Verification items for the finished model (mm, model axes). A direction names the side the tool comes from. Give positions to 0.01 mm unless a question says otherwise; leave off trailing zeros. Loops run counter-clockwise (first coordinate to the right, second up) from the corner with the lowest first, then second, coordinate; pieces in that order, holes last. Notation, with made-up numbers: M 19,31 L 76,31 A19 ccw 76,48 Z; hole C 82.5,18.5 d7. An arc over 180 degrees is marked long. Answer in a Markdown table with one row per item.
```python
from build123d import *

# Parameters (mm, degrees)
BOSS_EXTRUDE1_DEPTH         = 25.4
F_1_4_0_25_DIAMETER_HOLE1_D = 6.35


with BuildPart() as part:
    # Sketch1 → Boss-Extrude1 (new body)
    with BuildSketch(Plane(origin=(0, 0, 0), x_dir=(1, 0, 0), z_dir=(0, 1, 0))):
        Polygon((67.945, 0), (85.09, 0), (85.09, -5.08), (0, -5.08), (0, 0), (17.145, 0), (17.145, 5.08), (67.945, 5.08), align=None)
    extrude(amount=BOSS_EXTRUDE1_DEPTH)

    # 1/4 (0.25) Diameter Hole1 (through all)
    with Locations(Plane.XY.offset(5.08)):
        with Locations((5.715, 12.7), (79.375, 12.7)):
            Hole(F_1_4_0_25_DIAMETER_HOLE1_D / 2)


solid = part.part
```
Item 1: Scan lines: L1, parallel to X at y = 13.5, z = 1; L2, parallel to X at y = 14.5, z = -4.5 (3 decimals); L3, parallel to Z at x = 17, y = 15. Record each from-to range of solid material in increasing order. Write a range as [from, to].
Reported:
| item | result |
|---|---|
| L1 | x = [0, 2.64], [8.79, 76.3], [82.45, 85.09] |
| L2 | x = [17.145, 67.945] |
| L3 | z = [0, 5.08] |
Item 2: Sectioned sample at B-B (z = 1.5). Record the cut outline in (x, y) (3 decimals).
Reported:
| item | result |
|---|---|
| outline | M 0,0 L 85.09,0 L 85.09,25.4 L 0,25.4 Z; hole C 5.715,12.7 d6.35; hole C 79.375,12.7 d6.35 |
Item 3: Sectioned sample at D-D (x = 15). Record the cut outline in (y, z), and give its area (3 significant figures).
Reported:
| item | result |
|---|---|
| outline | M 0,0 L 25.4,0 L 25.4,5.08 L 0,5.08 Z |
| area | 129 mm^2 |
Item 4: Sectioned sample at A-A (y = 12.7). Record the cut outline in (x, z) (3 decimals), and give its area (3 significant figures).
Reported:
| item | result |
|---|---|
| outline | M 0,0 L 2.54,0 L 2.54,5.08 L 0,5.08 Z; M 8.89,0 L 17.145,0 L 17.145,-5.08 L 67.945,-5.08 L 67.945,0 L 76.2,0 L 76.2,5.08 L 8.89,5.08 Z; M 82.55,0 L 85.09,0 L 85.09,5.08 L 82.55,5.08 Z |
| area | 626 mm^2 |
Item 5: Go/stop test with flat-tipped pins: pin 1 (13.5 mm diameter, centred on x = 5, y = 15, fed in from -Z); pin 2 (1.5 mm diameter, centred on y = 7.5, z = -2, fed in from -X) (3 decimals). Record where each tip stops, or that it passes through.
Reported:
| item | result |
|---|---|
| pin 1 | stops at z = 0 |
| pin 2 | stops at x = 17.145 |
Item 6: Tool access check on faces 4 (the flat face through (17.145, 13, -3)), 5 (the flat face through (67.945, 13, -3)), 6 (the flat face through (0, 13, 3)). Record the directions out of +Z, -Z, +X, -X, +Y, -Y that give a thin tool (end or side, any length) a straight path to the whole face; none if there is none.
Reported:
| item | result |
|---|---|
| face 4 | -Z, -X, +Y, -Y |
| face 5 | -Z, +X, +Y, -Y |
| face 6 | +Z, -Z, -X, +Y, -Y |
Item 7: Sectioned sample at C-C (y = 17.75). Record the cut outline in (x, z) (3 decimals).
Reported:
| item | result |
|---|---|
| outline | M 0,0 L 17.145,0 L 17.145,-5.08 L 67.945,-5.08 L 67.945,0 L 85.09,0 L 85.09,5.08 L 0,5.08 Z |
Item 8: Release check for a two-part mould opening along Y. For faces 1 (the flat face through (43, 25.4, 1)), 2 (the flat face through (43, 0, 1)), 3 (the cylindrical face through (8.235, 10.768, 2.504)) record: released by +Y, released by -Y, zero draft, split by the parting line, or undercut.
Reported:
| item | result |
|---|---|
| face 1 | released by +Y |
| face 2 | released by -Y |
| face 3 | undercut |
